Model file for the job. Use its own axes, mm. Face numbers are marked on the shaded views. Coordinates: 2 decimals unless noted, no trailing zeros. Write each loop counter-clockwise with the first axis right and the second up, starting at its lowest first coordinate (ties: lowest second). Pieces come first, ordered by that corner, then holes. Notation, with made-up numbers: (9.25, 63) -> (47.25, 63) arc R13 cw to (47.25, 85) -> close; hole circle Ø10 at (-21, -33.75). An arc over 180 degrees is marked (long way). Answer as a JSON object with one key per item and string values. Group by question number.
from build123d import *

# Parameters (mm, degrees)
SKETCH1_W             = 9.525
SKETCH1_H             = 9.525
EXTRUDE1_DEPTH        = 28.575
F_4_40_TAPPED_HOLE1_D = 2.8448
F_4_40_TAPPED_HOLE2_D = 2.8448
CHAMFER1_SIZE         = 3.429


with BuildPart() as part:
    # Sketch1 → Extrude1 (new body)
    with BuildSketch(Plane.XY):
        Rectangle(SKETCH1_W, SKETCH1_H)
    extrude(amount=EXTRUDE1_DEPTH)

    # #4-40 Tapped Hole1 (through all)
    with Locations(Plane(origin=(0, 4.7625, 3.175), x_dir=(0, 0, 1), z_dir=(0, 1, 0))):
        with Locations((0, 0), (12.7, 0), (22.225, 0)):
            Hole(F_4_40_TAPPED_HOLE1_D / 2)

    # #4-40 Tapped Hole2 (through all)
    with Locations(Plane(origin=(-0.053117728, -4.7625, 20.699632052), x_dir=(0, 0, -1), z_dir=(0, -1, 0))):
        with Locations((0, 0), (11.1125, 0)):
            Hole(F_4_40_TAPPED_HOLE2_D / 2)

    # Chamfer1
    chamfer1_edges = [part.edges().sort_by_distance(p)[0] for p in [
        (-4.7625, 0, 0),
    ]]
    chamfer(chamfer1_edges, length=CHAMFER1_SIZE)


solid = part.part
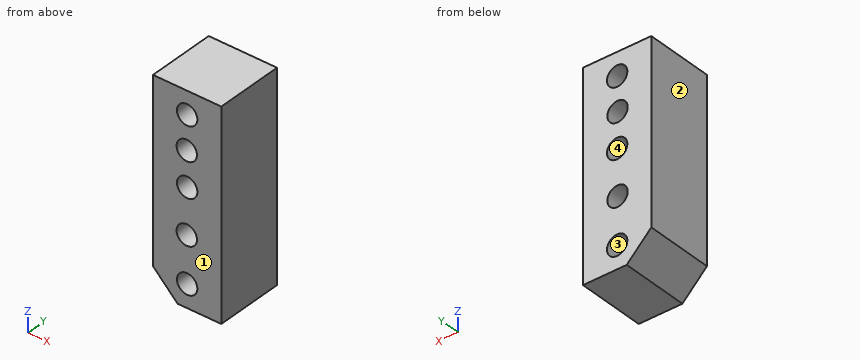
(1) Cut at D-D on x = -2.75. List the corners of the cut face in (y, z) (1 decimal), plus the area to 3 significant figures.
(2) Cut at C-C on y = -1. List the corners of the cut face in (x, z) (1 decimal), plus the area to 3 significant figures.
(3) Wall check: probe 1 along Z at (x, y) = (1, 0.25) (3 decimals); probe 2 along Z at (x, y) = (-1, -1.5) (3 decimals); probe 3 along X at (y, z) = (3.5, 3). Give the ranges that are in metal, low to high.
(4) Cut at B-B on x = 1. List the corners of the cut face in (y, z) (1 decimal), plus the area to 3 significant figures.
(5) Cut at A-A on z = 25.4. List the corners of the cut face in (x, y).
(6) Pin check, flat tip, straight feed: pin 1 (1.5 mm diameter, centred on x = -3.5, y = -1.5, fed in from -Z). Stop position of the tip, or through.
(7) Pull direction X, two halves, no side cores. Call the marked faces 1, 2, 3 and 4: released by +X, released by -X, zero draft, split by the parting line, or undercut.
Results found:
{
 "1": {"outline": "(-4.8, 1.4) -> (4.8, 1.4) -> (4.8, 28.6) -> (-4.8, 28.6) -> close", "area": "259 mm²"},
 "2": {"outline": "(-4.8, 3.4) -> (-1.3, 0) -> (4.8, 0) -> (4.8, 28.6) -> (-4.8, 28.6) -> close; hole circle Ø2.8 at (-0.1, 9.6); hole circle Ø2.8 at (-0.1, 20.7); hole circle Ø2.8 at (0, 3.2); hole circle Ø2.8 at (0, 15.9); hole circle Ø2.8 at (0, 25.4)", "area": "235 mm²"},
 "3": {"probe 1": "z = 0 to 2.163, 4.187 to 8.631, 10.543 to 14.863, 16.887 to 19.744, 21.656 to 24.388, 26.412 to 28.575", "probe 2": "z = 0 to 2.163, 4.187 to 8.526, 10.649 to 14.863, 16.887 to 19.638, 21.761 to 24.388, 26.412 to 28.575", "probe 3": "x = -4.33 to -1.41, 1.41 to 4.76"},
 "4": {"outline": "(-4.8, 0) -> (4.8, 0) -> (4.8, 2.2) -> (-4.8, 2.2) -> close; (-4.8, 4.2) -> (4.8, 4.2) -> (4.8, 8.6) -> (-4.8, 8.6) -> close; (-4.8, 10.5) -> (4.8, 10.5) -> (4.8, 14.9) -> (-4.8, 14.9) -> close; (-4.8, 16.9) -> (4.8, 16.9) -> (4.8, 19.7) -> (-4.8, 19.7) -> close; (-4.8, 21.7) -> (4.8, 21.7) -> (4.8, 24.4) -> (-4.8, 24.4) -> close; (-4.8, 26.4) -> (4.8, 26.4) -> (4.8, 28.6) -> (-4.8, 28.6) -> close", "area": "178 mm²"},
 "5": {"outline": "(-4.76, -4.76) -> (-1.42, -4.76) -> (-1.42, 4.76) -> (-4.76, 4.76) -> close; (1.42, -4.76) -> (4.76, -4.76) -> (4.76, 4.76) -> (1.42, 4.76) -> close"},
 "6": {"pin 1": "stops at z = 1.42"},
 "7": {"face 1": "zero draft", "face 2": "released by -X", "face 3": "undercut", "face 4": "undercut"}
}
